Read the model definition and answer for the solid it produces. Units are mm, in the model's axes. A direction names the side the tool comes from. Coordinates: 2 decimals unless noted, no trailing zeros. Loops run counter-clockwise (first coordinate to the right, second up) from the corner with the lowest first, then second, coordinate; pieces in that order, holes last.
Q1. Which of the six approach directions +Z, -Z, +X, -X, +Y, -Y give full straight-line access (tool end or side, diameter ignored) to faces 5 (the face through (35, 0, 9)), 6 (the face through (71.25, 11, 11))?
Q2. Section C-C (x = 58) is taken. Give the vertices of the cut face in (y, z), then the cut area to 3 significant figures.
Q3. Section D-D (z = 0.75) is taken. Give the vertices of the cut face in (x, y), then the cut area to 4 significant figures.
Q4. Section B-B (y = 9.5) is taken. Give the vertices of the cut face in (x, z), then the cut area to 4 significant figures.
Q5. Section A-A (z = 17.75) is taken. Give the vertices of the cut face in (x, y).
Q6. Straight lines are drawn through the part: line 1 (X direction, y = 3.5, z = 9.75); line 2 (X direction, y = 13, z = 16); line 3 (Y direction, x = 51.5, z = 9). For each, find the intervals that lie inside material, in ascending order.
Q7. The mould has two halves that part along X. Classify faces 1 (the face through (1.75, 3, 9)), 2 (the face through (0, 11, 9)), 3 (the face through (35, 11, -1)), 4 (the face through (36, 20, 9)): pulls with the +X half, pulls with the -X half, needs draft (parallel to the pull), parting line crosses it, or undercut.
Q8. A flat-ended cylindrical pin translates along its axis: P1, Ø1.5, axis at x = 55.5, y = 4, coming from the +Z side. Find the tip coordinate at first contact, or state that the pin passes through.
Autodesk Fusion 360 part; units mm, degrees
sketch "Sketch1" plane through (0, 0, 0) normal (0, 0, 1) x (1, 0, 0)
  line L0 (0, 0) -> (72, 0)
  line L1 (72, 0) -> (72, 21)
  line L2 (72, 21) -> (0, 21)
  line L3 (0, 21) -> (0, 0)
  line L4 (4.75, 20) -> (69.75, 20)
  line L5 (69.75, 20) -> (69.75, 1)
  line L6 (69.75, 1) -> (4.75, 1)
  line L7 (4.75, 1) -> (4.75, 20)
  line L8 (69.75, 20) -> (71.25, 20)
  line L9 (71.25, 20) -> (71.25, 1)
  line L10 (71.25, 1) -> (69.75, 1)
  line L11 (69.75, 1) -> (69.75, 20)
  line L12 (4.75, 20) -> (0.75, 20)
  line L13 (0.75, 20) -> (0.75, 1)
  line L14 (0.75, 1) -> (4.75, 1)
  line L15 (4.75, 1) -> (4.75, 20)
  line L16 (0.75, 18) -> (1.25, 18)
  line L17 (1.25, 18) -> (1.25, 3)
  line L18 (1.25, 3) -> (0.75, 3)
  line L19 (0.75, 3) -> (0.75, 18)
  line L20 (1.25, 14.5) -> (4.75, 14.5)
  line L21 (4.75, 14.5) -> (4.75, 6.5)
  line L22 (4.75, 6.5) -> (1.25, 6.5)
  line L23 (1.25, 6.5) -> (1.25, 14.5)
  line L24 (0.75, 20) -> (1.75, 20)
  line L25 (1.75, 20) -> (1.75, 18)
  line L26 (1.75, 18) -> (0.75, 18)
  line L27 (0.75, 18) -> (0.75, 20)
  line L28 (1.75, 18) -> (1.25, 18)
  line L29 (1.25, 18) -> (1.25, 17)
  line L30 (1.25, 17) -> (1.75, 17)
  line L31 (1.75, 17) -> (1.75, 18)
  line L32 (0.75, 3) -> (1.75, 3)
  line L33 (1.75, 3) -> (1.75, 1)
  line L34 (1.75, 1) -> (0.75, 1)
  line L35 (0.75, 1) -> (0.75, 3)
  line L36 (1.25, 3) -> (1.75, 3)
  line L37 (1.75, 3) -> (1.75, 4)
  line L38 (1.75, 4) -> (1.25, 4)
  line L39 (1.25, 4) -> (1.25, 3)
  line L40 (71.25, 18) -> (70.75, 18)
  line L41 (70.75, 18) -> (70.75, 3)
  line L42 (70.75, 3) -> (71.25, 3)
  line L43 (71.25, 3) -> (71.25, 18)
  line L44 (70.75, 14.5) -> (69.75, 14.5)
  line L45 (69.75, 14.5) -> (69.75, 6.5)
  line L46 (69.75, 6.5) -> (70.75, 6.5)
  line L47 (70.75, 6.5) -> (70.75, 14.5)
  line L48 (71.25, 20) -> (70.25, 20)
  line L49 (70.25, 20) -> (70.25, 18)
  line L50 (70.25, 18) -> (71.25, 18)
  line L51 (71.25, 18) -> (71.25, 20)
  line L52 (70.25, 18) -> (70.75, 18)
  line L53 (70.75, 18) -> (70.75, 17)
  line L54 (70.75, 17) -> (70.25, 17)
  line L55 (70.25, 17) -> (70.25, 18)
  line L56 (71.25, 3) -> (70.25, 3)
  line L57 (70.25, 3) -> (70.25, 1)
  line L58 (70.25, 1) -> (71.25, 1)
  line L59 (71.25, 1) -> (71.25, 3)
  line L60 (70.25, 3) -> (70.75, 3)
  line L61 (70.75, 3) -> (70.75, 4)
  line L62 (70.75, 4) -> (70.25, 4)
  line L63 (70.25, 4) -> (70.25, 3)
  dimension "d46" = 72
  dimension "d47" = 21
  dimension "d48" = 65
  dimension "d49" = 19
  dimension "d50" = 1
  dimension "d51" = 1.5
  dimension "d52" = 19
  dimension "d53" = 4
  dimension "d54" = 19
  dimension "d55" = 0.75
  dimension "d56" = 0.5
  dimension "d57" = 15
  dimension "d58" = 2
  dimension "d59" = 8
  dimension "d60" = 3.5
  dimension "d61" = 3.5
  dimension "d62" = 1
  dimension "d63" = 2
  dimension "d64" = 0.5
  dimension "d65" = 1
  dimension "d66" = 1
  dimension "d67" = 2
  dimension "d68" = 0.5
  dimension "d69" = 1
  dimension "d70" = 0.5
  dimension "d71" = 15
  dimension "d72" = 2
  dimension "d73" = 1
  dimension "d74" = 8
  dimension "d75" = 3.5
  dimension "d76" = 1
  dimension "d77" = 2
  dimension "d78" = 0.5
  dimension "d79" = 1
  dimension "d80" = 1
  dimension "d81" = 2
  dimension "d82" = 0.5
  dimension "d83" = 1
extrude "Extrude3" add sketch "Sketch1" against normal blind 1 contours L0 L1 L2 L3 | L4 L5 L6 L7 L11 L15 L21 L45 | L7 L12 L15 L17 L20 L25 L30 L31 | L5 L8 L11 L41 L44 L49 L54 L55 | L7 L15 L17 L20 L21 L22 L23 | L12 L13 L16 L24 L25 L26 L27 L28 | L5 L11 L41 L44 L45 L46 L47 | L8 L9 L40 L48 L49 L50 L51 L52 | L7 L14 L15 L17 L22 L33 L37 L38 | L13 L16 L17 L18 L19 L23 L26 L29 L32 L39 | L17 L26 L28 L29 L30 L31 | L5 L10 L11 L41 L46 L57 L62 L63 | L9 L40 L41 L42 L43 L47 L50 L53 L56 L61 | L41 L50 L52 L53 L54 L55 | L13 L14 L18 L32 L33 L34 L35 L36 | L17 L32 L36 L37 L38 L39 | L9 L10 L42 L56 L57 L58 L59 L60 | L41 L56 L60 L61 L62 L63
extrude "Extrude4" add sketch "Sketch1" along normal blind 19 contours L0 L1 L2 L3 | L12 L13 L16 L24 L25 L26 L27 L28 | L8 L9 L40 L48 L49 L50 L51 L52 | L17 L26 L28 L29 L30 L31 | L41 L50 L52 L53 L54 L55 | L13 L14 L18 L32 L33 L34 L35 L36 | L17 L32 L36 L37 L38 L39 | L9 L10 L42 L56 L57 L58 L59 L60 | L41 L56 L60 L61 L62 L63
extrude "Extrude5" add sketch "Sketch1" along normal blind 3 contours L13 L16 L17 L18 L19 L23 L26 L29 L32 L39 | L9 L40 L41 L42 L43 L47 L50 L53 L56 L61
Numbers:
1. face 5: +Z, -Z, +X, -X, -Y
1. face 6: +Z
2. outline: (0, -1) - (21, -1) - (21, 19) - (20, 19) - (20, 0) - (1, 0) - (1, 19) - (0, 19) - close
2. area: 59.0 mm2
3. outline: (0, 0) - (72, 0) - (72, 21) - (0, 21) - close; hole (1.25, 4) - (1.75, 4) - (1.75, 1) - (70.25, 1) - (70.25, 4) - (70.75, 4) - (70.75, 17) - (70.25, 17) - (70.25, 20) - (1.75, 20) - (1.75, 17) - (1.25, 17) - close
3. area: 197.5 mm2
4. outline: (0, -1) - (72, -1) - (72, 19) - (71.25, 19) - (71.25, 3) - (70.75, 3) - (70.75, 0) - (1.25, 0) - (1.25, 3) - (0.75, 3) - (0.75, 19) - (0, 19) - close
4. area: 103.5 mm2
5. outline: (0, 0) - (72, 0) - (72, 21) - (0, 21) - close; hole (0.75, 3) - (1.25, 3) - (1.25, 4) - (1.75, 4) - (1.75, 1) - (70.25, 1) - (70.25, 4) - (70.75, 4) - (70.75, 3) - (71.25, 3) - (71.25, 18) - (70.75, 18) - (70.75, 17) - (70.25, 17) - (70.25, 20) - (1.75, 20) - (1.75, 17) - (1.25, 17) - (1.25, 18) - (0.75, 18) - close
6. line 1: x = 0 to 0.75, 1.25 to 1.75, 70.25 to 70.75, 71.25 to 72
6. line 2: x = 0 to 0.75, 71.25 to 72
6. line 3: y = 0 to 1, 20 to 21
7. face 1: undercut
7. face 2: pulls with the -X half
7. face 3: needs draft
7. face 4: undercut
8. P1: stops at z = 0
